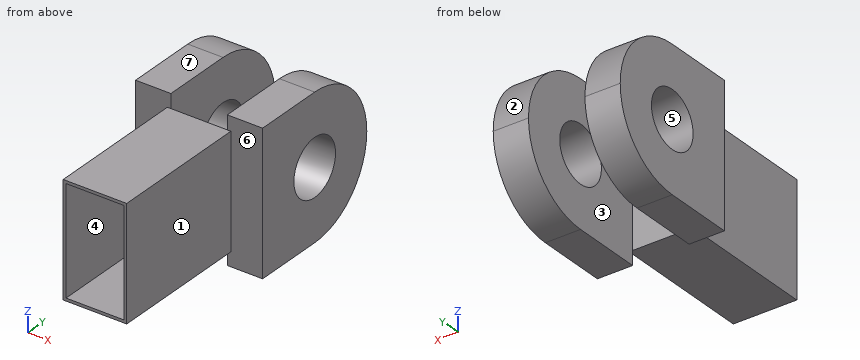
from build123d import *

# Parameters (mm, degrees)
SKETCH1_W           = 9
SKETCH1_H           = 16
BOSS_EXTRUDE1_DEPTH = 20
SKETCH2_W           = 8.2
SKETCH2_H           = 15.2
CUT_EXTRUDE1_DEPTH  = 18
SKETCH4_W           = 5
SKETCH4_H           = 20
BOSS_EXTRUDE2_DEPTH = 20
SKETCH5_R           = 4
CUT_EXTRUDE2_DEPTH  = 45.988887517
FILLET1_R           = 10


with BuildPart() as part:
    # Sketch1 → Boss-Extrude1 (new body)
    with BuildSketch(Plane(origin=(0, 0, 0), x_dir=(1, 0, 0), z_dir=(0, 1, 0))):
        Rectangle(SKETCH1_W, SKETCH1_H)
    extrude(amount=BOSS_EXTRUDE1_DEPTH)

    # Sketch2 → Cut-Extrude1 (cut)
    with BuildSketch(Plane.XZ):
        Rectangle(SKETCH2_W, SKETCH2_H)
    extrude(amount=-CUT_EXTRUDE1_DEPTH, mode=Mode.SUBTRACT)

    # Sketch4 → Boss-Extrude2 (add)
    with BuildSketch(Plane(origin=(0, 20, 0), x_dir=(1, 0, 0), z_dir=(0, 1, 0))):
        with Locations((6.5, 0)):
            Rectangle(SKETCH4_W, SKETCH4_H)
        with Locations((-6.5, 0)):
            Rectangle(SKETCH4_W, SKETCH4_H)
    extrude(amount=BOSS_EXTRUDE2_DEPTH)

    # Sketch5 → Cut-Extrude2 (cut, through all)
    with BuildSketch(Plane(origin=(9, 0, 0), x_dir=(0, 0, -1), z_dir=(1, 0, 0))):
        with Locations((0, 30)):
            Circle(SKETCH5_R)
    extrude(amount=-CUT_EXTRUDE2_DEPTH, mode=Mode.SUBTRACT)

    # Fillet1
    fillet1_edges = [part.edges().sort_by_distance(p)[0] for p in [
        (6.5, 40, 10),
        (6.5, 40, -10),
        (-6.5, 40, -10),
        (-6.5, 40, 10),
    ]]
    fillet(fillet1_edges, radius=FILLET1_R - 0.0001)  # a hair under: the kernel refuses the full size


solid = part.part
Read the model definition and answer for the solid it produces. Units are mm, in the model's axes. Face numbers are marked on the shaded views. A direction names the side the tool comes from. Round coordinates to 2 decimals unless told otherwise and drop trailing zeros. Loops run counter-clockwise (first coordinate to the right, second up) from the corner with the lowest first, then second, coordinate; pieces in that order, holes last.
Q1. Which of the six approach directions +Z, -Z, +X, -X, +Y, -Y give full straight-line access (tool end or side, diameter ignored) to the marked faces 1, 2 and 3?
Q2. Determine the mould class of the marked faces 4, 5, 6 and 7 for opening direction Z: released by +Z, released by -Z, zero draft, split by the parting line, or undercut.
Q3. Each of these flat-tipped pins is pushed along its axis until it touches: pin 1 (4 mm diameter, centred on y = 17, z = 5, fed in from -X); pin 2 (4 mm diameter, centred on x = 7.5, z = -1.5, fed in from -Y); pin 3 (4 mm diameter, centred on x = 7, z = -3, fed in from +Y); pin 4 (6 mm diameter, centred on y = 32, z = -2.5, fed in from +X). Where does it stop, or does it pass through?
Q4. Section B-B on y = 23 is taken. Write down the section's boundary in (x, z).
Q5. Section C-C on z = -2.5 is taken. Write down the section's boundary in (x, y), and give its area (3 significant figures).
Q6. Consider probe 1 along Y at (x, z) = (6.3, 0); probe 2 along X at (y, z) = (37.5, 6.25); probe 3 along Z at (x, y) = (2.75, 7). Determine where each line is inside the solid, lowest interval first.
Q7. Section D-D on y = 4.5 is taken. Write down the section's boundary in (x, z).
Output:
1. face 1: +Z, -Z, +X, -Y
1. face 2: +Z, +X, -X, +Y
1. face 3: +Z, -Z, +Y
2. face 4: undercut
2. face 5: undercut
2. face 6: zero draft
2. face 7: released by +Z
3. pin 1: stops at x = -4.5
3. pin 2: stops at y = 20
3. pin 3: stops at y = 39.95
3. pin 4: stops at x = 9
4. outline: (-9, -10) - (-4, -10) - (-4, 10) - (-9, 10) - close; (4, -10) - (9, -10) - (9, 10) - (4, 10) - close
5. outline: (-9, 20) - (-4.5, 20) - (-4.5, 0) - (-4.1, 0) - (-4.1, 18) - (4.1, 18) - (4.1, 0) - (4.5, 0) - (4.5, 20) - (9, 20) - (9, 26.88) - (4, 26.88) - (4, 20) - (-4, 20) - (-4, 26.88) - (-9, 26.88) - close; (-9, 33.12) - (-4, 33.12) - (-4, 39.68) - (-9, 39.68) - close; (4, 33.12) - (9, 33.12) - (9, 39.68) - (4, 39.68) - close
5. area: 167 mm2
6. probe 1: y = 20 to 26, 34 to 40
6. probe 2: x = -9 to -4, 4 to 9
6. probe 3: z = -8 to -7.6, 7.6 to 8
7. outline: (-4.5, -8) - (4.5, -8) - (4.5, 8) - (-4.5, 8) - close; hole (-4.1, -7.6) - (4.1, -7.6) - (4.1, 7.6) - (-4.1, 7.6) - close
